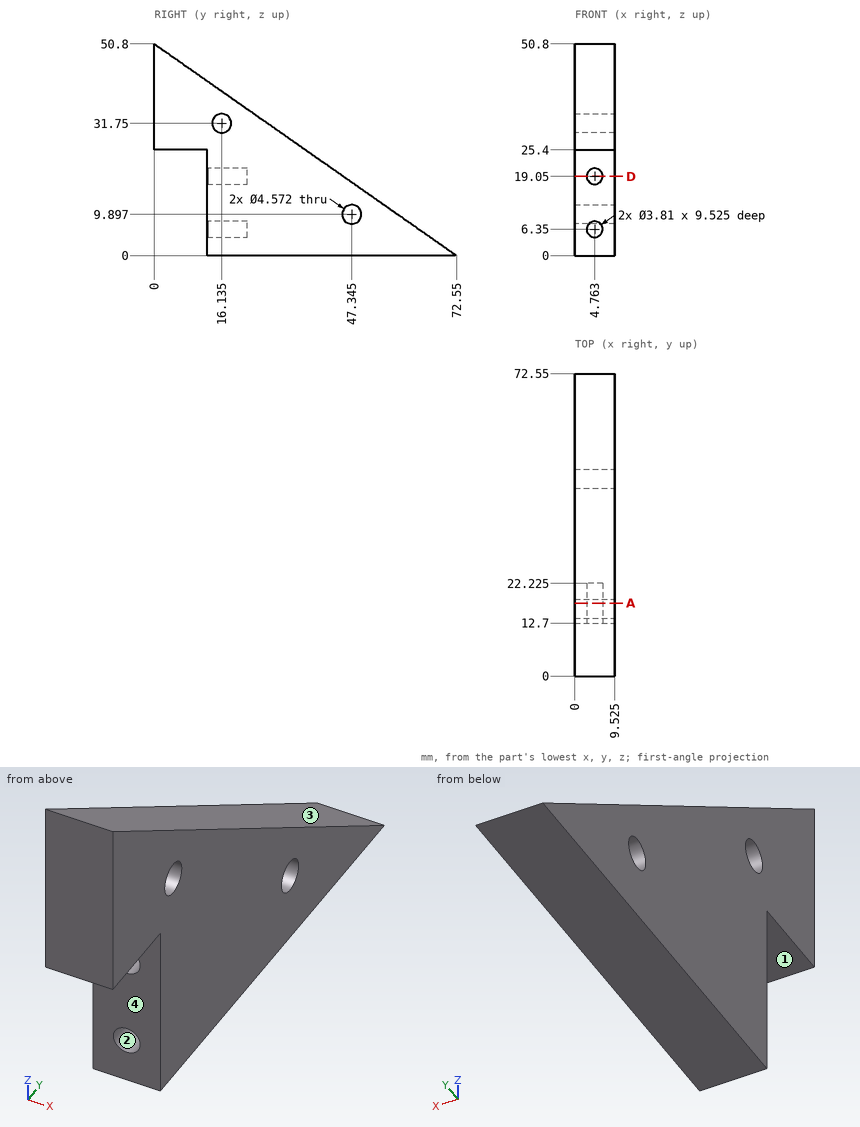
Part print with two shaded views. Sizes in mm from the minimum x, y, z corner. Round coordinates to 2 decimals unless told otherwise and drop trailing zeros. Order: outer loops, then holes, each group sorted by start corner. A loop starts at its lowest first (then second) coordinate and runs counter-clockwise, first axis right, second up. Notation, with made-up numbers: M 22.25,-17.75 L 34.25,-17.75 A30 cw 34.25,19.25 Z; hole C 2,49.25 d10. An arc over 180 degrees is marked long. Use CSV: the item, a comma, the result in double quotes.
Item 1: Saw through at D-D (z = 19.05). List the corners of the cut face in (x, y) (1 decimal).
Worked answers:
outline,"M 0,12.7 L 2.9,12.7 L 2.9,22.2 L 6.7,22.2 L 6.7,12.7 L 9.5,12.7 L 9.5,45.3 L 0,45.3 Z"
Item 2: Pin check, flat tips, straight feed: pin 1 (1.1 mm diameter, centred on x = 5.5, z = 19, fed in from -Y) (1 decimal); pin 2 (5 mm diameter, centred on x = 6.5, z = 9.5, fed in from -Y); pin 3 (4.5 mm diameter, centred on x = 4.76, z = 19.05, fed in from +Y) (1 decimal). Stop position of each tip, or through.
Worked answers:
pin 1,"y = 22.2"
pin 2,"y = 12.7"
pin 3,"y = 48.6"
Item 3: Pull direction Z, two halves, no side cores. Call the marked faces 1, 2, 3 and 4: released by +Z, released by -Z, zero draft, split by the parting line, or undercut.
Worked answers:
face 1,"released by -Z"
face 2,"undercut"
face 3,"released by +Z"
face 4,"zero draft"
Item 4: Probe probe 1 along X at (y, z) = (18, 6.35) (1 decimal); probe 2 along Z at (x, y) = (4.75, 20.5) (1 decimal); probe 3 along Z at (x, y) = (2.75, 15) (1 decimal). List the from-to ranges inside material, lowest first.
Worked answers:
probe 1,"0 to 2.9, 6.7 to 9.5"
probe 2,"0 to 4.4, 8.3 to 17.1, 21 to 36.4"
probe 3,"0 to 29.8, 33.7 to 40.3"
Item 5: Saw through at A-A (y = 17.5). State how many separate pieces and enclosed holes the cut face has.
Worked answers:
separate pieces,"2"
enclosed holes,"2"
